from build123d import *

# Parameters (mm, degrees)
F0_W     = 200
F0_H     = 35
F1_DEPTH = 5
F2_R     = 4
F3_DEPTH = 10


with BuildPart() as f1:
    # F0 (on Front) → F1 (new body)
    with BuildSketch(Plane.XZ):
        Rectangle(F0_W, F0_H)
    extrude(amount=F1_DEPTH)

    # F2 (on face) → F3 (join)
    with BuildSketch(Plane.XZ.offset(5)):
        with Locations((-75, 0)):
            Circle(F2_R)
        Circle(F2_R)
        with Locations((75, 0)):
            Circle(F2_R)
    extrude(amount=F3_DEPTH)


solid = f1.part
Work out the finished part from the listing and answer in its coordinate system (mm). A direction names the side the tool comes from. Give positions to 0.01 mm unless a question says otherwise; leave off trailing zeros. Order: outer loops, then holes, each group sorted by start corner. A loop starts at its lowest first (then second) coordinate and runs counter-clockwise, first axis right, second up. Notation, with made-up numbers: (-10, -13.5) -> (34, -13.5) arc R25 cw to (34, 17.5) -> close; hole circle Ø2 at (60.5, 77.5). An arc over 180 degrees is marked (long way). Answer as a JSON object with one key per item and string values. Group by question number.
1. Consider line 1 along X through (y, z) = (-13, 3); line 2 along X through (y, z) = (-11, 2); line 3 along Y through (x, z) = (8, -9.5). Determine where each line is inside the solid, lowest interval first. Write a range as [from, to].
2. Section A-A on x = 0 is taken. Determine the outline of the cut face in (y, z).
3. Section D-D on x = 54.5 is taken. Determine the outline of the cut face in (y, z).
4. The mould has two halves that part along X. Classify faces 3 (the cylindrical face through (-79, -10, 0)), 4 (the flat face through (0, -15, 0)), 5 (the flat face through (100, -2, 0)): released by +X, released by -X, zero draft, split by the parting line, or undercut.
5. Section B-B on z = 0 is taken. Determine the outline of the cut face in (x, y).
6. A tool of negligible diameter and unlimited length cuts with its end or side. For faces 1 (the flat face through (-75, -15, 0)), 2 (the cylindrical face through (-0.867, -9.93, -3.905)), from which of +Z, -Z, +X, -X, +Y, -Y can it reach the whole face along a straight path? Write none if from no direction.
7. Section C-C on y = -12 is taken. Determine the outline of the cut face in (x, z), plus the area to 3 significant figures.
8. Flat-ended cylindrical pins translate along their axes: pin 1 Ø8 at (y, z) = (-5.5, 9.5) entering from -X; pin 2 Ø10.5 at (x, z) = (11, -1.5) entering from -Y. Find the tip coordinate at first contact, or state that the pin passes through.
Result sheet:
{
 "1": {"line 1": "x = [-77.65, -72.35], [-2.65, 2.65], [72.35, 77.65]", "line 2": "x = [-78.46, -71.54], [-3.46, 3.46], [71.54, 78.46]", "line 3": "y = [-5, 0]"},
 "2": {"outline": "(-15, -4) -> (-5, -4) -> (-5, -17.5) -> (0, -17.5) -> (0, 17.5) -> (-5, 17.5) -> (-5, 4) -> (-15, 4) -> close"},
 "3": {"outline": "(-5, -17.5) -> (0, -17.5) -> (0, 17.5) -> (-5, 17.5) -> close"},
 "4": {"face 3": "undercut", "face 4": "zero draft", "face 5": "released by +X"},
 "5": {"outline": "(-100, -5) -> (-79, -5) -> (-79, -15) -> (-71, -15) -> (-71, -5) -> (-4, -5) -> (-4, -15) -> (4, -15) -> (4, -5) -> (71, -5) -> (71, -15) -> (79, -15) -> (79, -5) -> (100, -5) -> (100, 0) -> (-100, 0) -> close"},
 "6": {"face 1": "+Z, -Z, +X, -X, -Y", "face 2": "-Y"},
 "7": {"outline": "circle Ø8 at (-75, 0); circle Ø8 at (0, 0); circle Ø8 at (75, 0)", "area": "151 mm^2"},
 "8": {"pin 1": "stops at x = -100", "pin 2": "stops at y = -5"}
}
